Source: CAD feature listing. Evaluate the final solid. Frame: model axes, mm. A direction names the side the tool comes from. Coordinates: 2 decimals unless noted, no trailing zeros. Order: outer loops, then holes, each group sorted by start corner. A loop starts at its lowest first (then second) coordinate and runs counter-clockwise, first axis right, second up. Notation, with made-up numbers: (-29, 72) - (20, 72) arc R29 cw to (20, 109) - close; hole circle Ø5 at (31, 11.5). An arc over 180 degrees is marked (long way). One line per question, with ' | ' between items. Start each with the question number.
(1) Line query: line 1 along Y through (x, z) = (-0.25, 1.35); line 2 along X through (y, z) = (-3, 1.55); line 3 along X through (y, z) = (-1.25, 1.65). Output: solid intervals per line, ascending.
(2) Section A-A (y = 0). Return the cut outline in (x, z) (3 decimals).
(3) Section D-D (x = 1.75). Return the cut outline in (y, z).
(4) Section C-C (x = 7.5). Return the cut outline in (y, z).
(5) Draft query along X for faces 1 (the flat face through (-7, 2, 3)), 2 (the flat face through (0, 3, 1.3)). Return one class per face: +X half, -X half, draft (parallel to the pull), parting line (faces both ways), or undercut.
(6) Contact query for flat-ended pins moving along their axis: P1, Ø2, axis at x = -4.5, y = 2, coming from the -Z side; P2, Ø0.8, axis at x = -1.5, y = -3, coming from the +Z side; P3, Ø0.8, axis at x = -1.5, y = 2, coming from the +Z side. Output: stop coordinate, or through.
(7) Section B-B (z = 2.1). Return the cut outline in (x, y) (3 decimals), then the cut area to 3 significant figures.
(8) Access query for faces 3 (the flat face through (0, 0, 2.3)), 4 (the flat face through (0, -3, 1.3)), 5 (the flat face through (0, 4.5, 1)). Directions: +Z, -Z, +X, -X, +Y, -Y. A direction counts if a zero-diameter tool reaches every point of the face in a straight line with its end or side. Return the directions, or none.
from build123d import *

# Parameters (mm, degrees)
F0_W     = 20
F0_H     = 9
F1_DEPTH = 3
F3_DEPTH = 3.25
F4_R     = 1.85
F5_DEPTH = 25


with BuildPart() as f1:
    # F0 (on Top) → F1 (new body)
    with BuildSketch(Plane.XY):
        Rectangle(F0_W, F0_H)
    extrude(amount=F1_DEPTH)

    # F2 (on Right) → F3 (cut, symmetric)
    with BuildSketch(Plane.YZ):
        Polygon((4.5, 3), (0, 3), (-4.5, 3), (-4.5, 2.3), (-3.5, 2.3), (-3.5, 1.3), (-2.5, 1.3), (-2.5, 2.3), (-1.5, 2.3), (-1.5, 1.3), (-0.5, 1.3), (-0.5, 2.3), (0, 2.3), (0.5, 2.3), (0.5, 1.3), (1.5, 1.3), (1.5, 2.3), (2.5, 2.3), (2.5, 1.3), (3.5, 1.3), (3.5, 2.3), (4.5, 2.3), align=None)
    extrude(amount=F3_DEPTH, both=True, mode=Mode.SUBTRACT)

    # F4 (on face) → F5 (cut)
    with BuildSketch(Plane.XY.offset(3)):
        with Locations((-6.625, 0)):
            Circle(F4_R)
        with Locations((6.625, 0)):
            Circle(F4_R)
    extrude(amount=-F5_DEPTH, mode=Mode.SUBTRACT)


solid = f1.part
Response values:
1) line 1: y = -4.5 to -3.5, -2.5 to -1.5, -0.5 to 0.5, 1.5 to 2.5, 3.5 to 4.5 | line 2: x = -10 to -3.25, 3.25 to 10 | line 3: x = -10 to -7.99, -5.26 to -3.25, 3.25 to 5.26, 7.99 to 10
2) outline: (-10, 0) - (-8.475, 0) - (-8.475, 3) - (-10, 3) - close; (-4.775, 0) - (4.775, 0) - (4.775, 3) - (3.25, 3) - (3.25, 2.3) - (-3.25, 2.3) - (-3.25, 3) - (-4.775, 3) - close; (8.475, 0) - (10, 0) - (10, 3) - (8.475, 3) - close
3) outline: (-4.5, 0) - (4.5, 0) - (4.5, 2.3) - (3.5, 2.3) - (3.5, 1.3) - (2.5, 1.3) - (2.5, 2.3) - (1.5, 2.3) - (1.5, 1.3) - (0.5, 1.3) - (0.5, 2.3) - (-0.5, 2.3) - (-0.5, 1.3) - (-1.5, 1.3) - (-1.5, 2.3) - (-2.5, 2.3) - (-2.5, 1.3) - (-3.5, 1.3) - (-3.5, 2.3) - (-4.5, 2.3) - close
4) outline: (-4.5, 0) - (-1.63, 0) - (-1.63, 3) - (-4.5, 3) - close; (1.63, 0) - (4.5, 0) - (4.5, 3) - (1.63, 3) - close
5) face 1: draft | face 2: undercut
6) P1: stops at z = 0 | P2: stops at z = 1.3 | P3: stops at z = 2.3
7) outline: (-10, -4.5) - (10, -4.5) - (10, 4.5) - (-10, 4.5) - close; hole circle Ø3.7 at (-6.625, 0); hole (-3.25, -3.5) - (3.25, -3.5) - (3.25, -2.5) - (-3.25, -2.5) - close; hole (-3.25, -1.5) - (3.25, -1.5) - (3.25, -0.5) - (-3.25, -0.5) - close; hole (-3.25, 0.5) - (3.25, 0.5) - (3.25, 1.5) - (-3.25, 1.5) - close; hole (-3.25, 2.5) - (3.25, 2.5) - (3.25, 3.5) - (-3.25, 3.5) - close; hole circle Ø3.7 at (6.625, 0) | area: 132 mm²
8) face 3: +Z, +Y, -Y | face 4: +Z | face 5: +Z, -Z, +X, -X, +Y
